Verification items for the finished model (mm, model axes). Coordinates: 2 decimals unless noted, no trailing zeros. Order: outer loops, then holes, each group sorted by start corner. A loop starts at its lowest first (then second) coordinate and runs counter-clockwise, first axis right, second up. Notation, with made-up numbers: (-13.5, -17.75) -> (8.5, -17.75) arc R15 ccw to (8.5, -5.75) -> close; hole circle Ø1 at (-9.75, 17). An arc over 180 degrees is marked (long way). Use CSV: the item, a comma, the result in double quotes. Start each with the question number.
1) Sectioned sample at A-A on z = 45.5. Record the boundary of the cut face in (x, y).
2) Sectioned sample at B-B on x = 64.5. Record the boundary of the cut face in (y, z) (3 decimals).
3) Sectioned sample at C-C on x = -40. Record the boundary of the cut face in (y, z), then the cut area to 3 significant figures.
4) Scan lines: line 1 along X through (y, z) = (0.5, 45.5); line 2 along Z through (x, y) = (-64.5, 0.65) (3 decimals); line 3 along Z through (x, y) = (-63.5, 0.75). Record each from-to range of solid material in increasing order.
Autodesk Inventor part; units mm, degrees
ref_plane "YZ Plane" through (0, 0, 0) normal (1, 0, 0) x (0, 1, 0)
ref_plane "XZ Plane" through (0, 0, 0) normal (0, 1, 0) x (-1, 0, 0)
ref_plane "XY Plane" through (0, 0, 0) normal (0, 0, 1) x (1, 0, 0)
sketch "Sketch1" plane through (0, 0, 0) normal (0, 1, 0) x (-1, 0, 0)
  line L0 (64.5, 64.625) -> (-64.5, 64.625) construction
  line L1 (-64.5, 64.625) -> (-64.5, -64.625) construction
  line L2 (-64.5, -64.625) -> (62.5, -64.625) construction
  line L3 (64.5, -62.625) -> (64.5, 64.625) construction
  line L4 (64.5, 64.625) -> (-64.5, -64.625) construction
  line L5 (-64.5, 64.625) -> (64.5, -64.625) construction
  line L6 (68.5, 70.5) -> (-68.5, 70.5)
  line L7 (-70.5, 68.5) -> (-70.5, -68.5)
  line L8 (-68.5, -70.5) -> (68.5, -70.5)
  line L9 (70.5, -68.5) -> (70.5, 68.5)
  line L10 (70.5, 70.5) -> (-70.5, -70.5) construction
  line L11 (-70.5, 70.5) -> (70.5, -70.5) construction
  arc A0 (62.5, -64.625) -> (64.5, -62.625) centre (62.5, -62.625) ccw
  arc A1 (70.5, 68.5) -> (68.5, 70.5) centre (68.5, 68.5) ccw
  arc A2 (68.5, -70.5) -> (70.5, -68.5) centre (68.5, -68.5) ccw
  arc A3 (-70.5, -68.5) -> (-68.5, -70.5) centre (-68.5, -68.5) ccw
  arc A4 (-68.5, 70.5) -> (-70.5, 68.5) centre (-68.5, 68.5) ccw
  point P0 (0, 0)
  dimension "d0" = 129
  dimension "d1" = 129.25
  dimension "d2" = 141
  dimension "d3" = 141
  dimension "d4" = 2
extrude "Extrusion1" add sketch "Sketch1" along normal blind 2
hole "Hole1" at (64.5, 0, -64.625) at (64.5, 0, 64.625) at (-64.5, 0, -64.625) at (-64.5, 0, 64.625) direction (0, 1, 0) diameter 4 end through all
sketch "Sketch2" plane through (0, 2, 0) normal (0, 1, 0) x (1, 0, 0)
  circle A0 centre (-64.5, 64.625) radius 2 construction
  circle A1 centre (64.5, 64.625) radius 2 construction
  circle A2 centre (64.5, -64.625) radius 2 construction
  circle A3 centre (-64.5, -64.625) radius 2 construction
  arc A4 (68.5, -70.5) -> (70.5, -68.5) centre (68.5, -68.5) ccw construction
  line L0 (70.5, -68.5) -> (70.5, 68.5) construction
  arc A5 (70.5, 68.5) -> (68.5, 70.5) centre (68.5, 68.5) ccw construction
  line L1 (68.5, 70.5) -> (-68.5, 70.5) construction
  arc A6 (-68.5, 70.5) -> (-70.5, 68.5) centre (-68.5, 68.5) ccw construction
  line L2 (-70.5, 68.5) -> (-70.5, -68.5) construction
  arc A7 (-70.5, -68.5) -> (-68.5, -70.5) centre (-68.5, -68.5) ccw construction
  line L3 (-68.5, -70.5) -> (68.5, -70.5) construction
  line L4 (70.5, -68.5) -> (70.5, 68.5) construction
  line L5 (70.5, -45.5) -> (-70.5, -45.5) construction
  line L6 (-70.5, 68.5) -> (-70.5, -68.5) construction
  line L7 (0, -45.5) -> (-40, -45.5) construction
  line L8 (-40, -45.5) -> (0, -45.5) construction
  line L9 (0, -45.5) -> (40, -45.5) construction
  point P0 (0, 0)
  dimension "d14" = 25
  dimension "d15" = 40
  dimension "d16" = 40
hole "Hole2" at (-40, 2, 45.5) at (40, 2, 45.5) direction (0, -1, 0) diameter 4 end through all countersink diameter 6 countersink angle 90
properties part number "plate_f16"
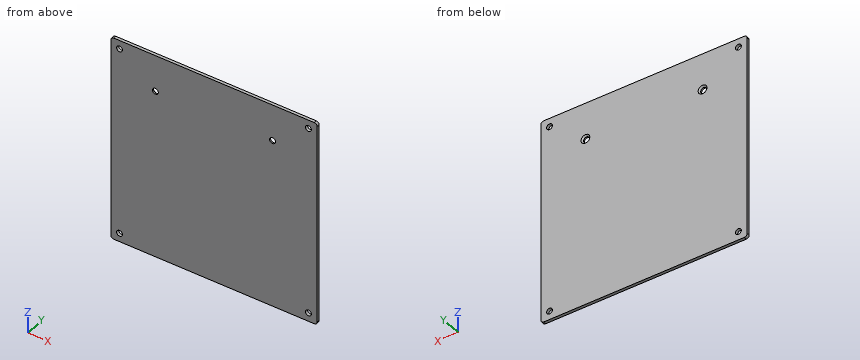
Answers follow:
1,outline,"(-70.5, 0) -> (-42, 0) -> (-42, 1) -> (-43, 2) -> (-70.5, 2) -> close; (-38, 0) -> (38, 0) -> (38, 1) -> (37, 2) -> (-37, 2) -> (-38, 1) -> close; (42, 0) -> (70.5, 0) -> (70.5, 2) -> (43, 2) -> (42, 1) -> close"
2,outline,"(0, -70.5) -> (2, -70.5) -> (2, -66.625) -> (0, -66.625) -> close; (0, -62.625) -> (2, -62.625) -> (2, 62.625) -> (0, 62.625) -> close; (0, 66.625) -> (2, 66.625) -> (2, 70.5) -> (0, 70.5) -> close"
3,outline,"(0, -70.5) -> (2, -70.5) -> (2, 42.5) -> (1, 43.5) -> (0, 43.5) -> close; (0, 47.5) -> (1, 47.5) -> (2, 48.5) -> (2, 70.5) -> (0, 70.5) -> close"
3,area,"273 mm²"
4,line 1,"x = -70.5 to -42, -38 to 38, 42 to 70.5"
4,line 2,"z = -70.5 to -66.625, -62.625 to 62.625, 66.625 to 70.5"
4,line 3,"z = -70.5 to -66.36, -62.89 to 62.89, 66.36 to 70.5"
